Can you work these out from the drawing? Everything is in mm from the part's minimum corner. A direction names the side the tool comes from. Give positions to 0.01 mm unless a question says otherwise; leave off trailing zeros. Write each loop counter-clockwise with the first axis right and the second up, starting at its lowest first coordinate (ties: lowest second). Pieces come first, ordered by that corner, then holes. Notation, with made-up numbers: (-22.5, 34) - (-6.5, 34) arc R27 ccw to (-6.5, 65) - close; hole circle Ø8 at (-27.75, 12). An arc over 180 degrees is marked (long way). Answer in a Markdown table with one row per item.
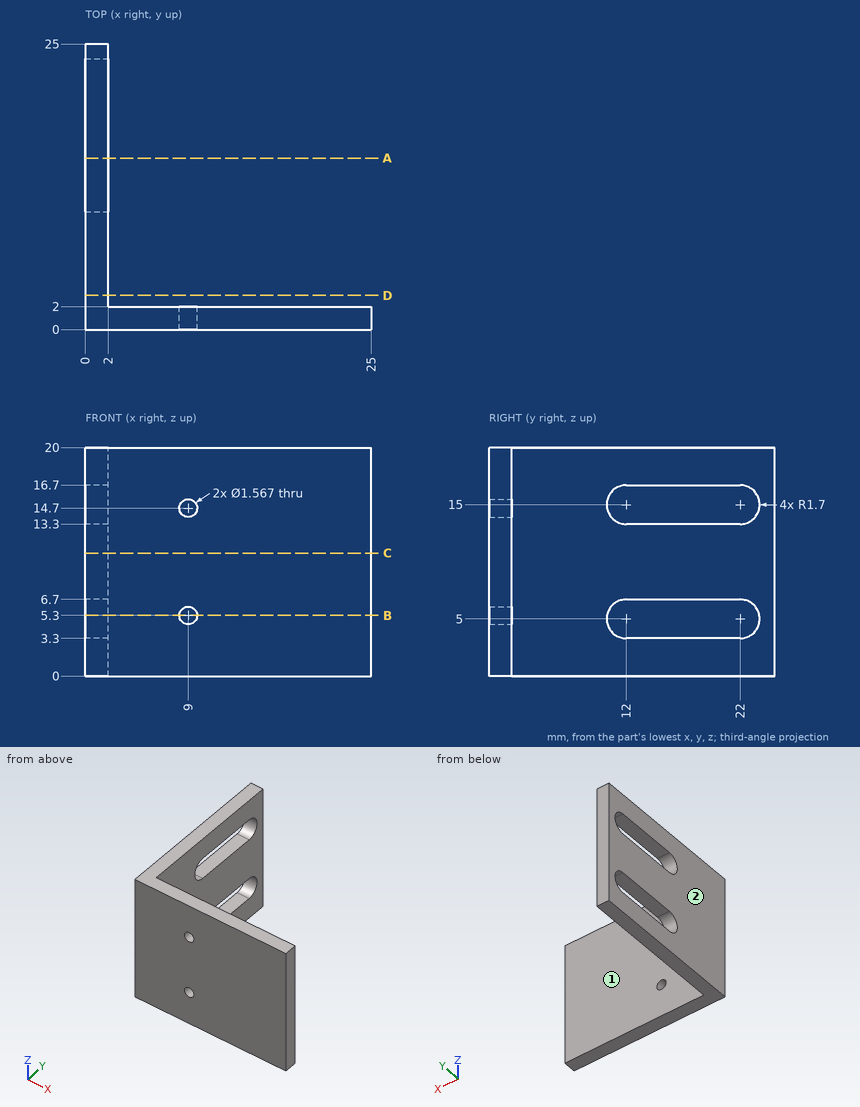
1) Will these pins go through, and if not, where does the flat tip stop? P1, Ø6, axis at x = 17.5, z = 12, coming from the +Y side; P2, Ø2, axis at x = 9, z = 5.3, coming from the -Y side; P3, Ø6, axis at y = 14, z = 6, coming from the +X side.
Check values:
| item | result |
|---|---|
| P1 | stops at y = 2 |
| P2 | stops at y = 0 |
| P3 | stops at x = 2 |
2) Imagine slicing it at B-B (z = 5.3). List the corners of the cut face in (x, y) for me, then the cut area to 3 significant figures.
Check values:
| item | result |
|---|---|
| outline | (0, 0) - (8.22, 0) - (8.22, 2) - (2, 2) - (2, 10.33) - (0, 10.33) - close; (0, 23.67) - (2, 23.67) - (2, 25) - (0, 25) - close; (9.78, 0) - (25, 0) - (25, 2) - (9.78, 2) - close |
| area | 66.2 mm2 |
3) Imagine slicing it at D-D (y = 3). List the corners of the cut face in (x, z) for me.
Check values:
| item | result |
|---|---|
| outline | (0, 0) - (2, 0) - (2, 20) - (0, 20) - close |
4) Imagine slicing it at A-A (y = 15). List the corners of the cut face in (x, z) for me.
Check values:
| item | result |
|---|---|
| outline | (0, 0) - (2, 0) - (2, 3.3) - (0, 3.3) - close; (0, 6.7) - (2, 6.7) - (2, 13.3) - (0, 13.3) - close; (0, 16.7) - (2, 16.7) - (2, 20) - (0, 20) - close |
5) If I drill on line 1 (Z direction, x = 9, y = 1.1); line 2 (X direction, y = 1.2, z = 5.3); line 3 (Y direction, x = 4.5, z = 5), over which ranges is the centre line in solid material (lowest first)?
Check values:
| item | result |
|---|---|
| line 1 | z = 0 to 4.52, 6.08 to 13.92, 15.48 to 20 |
| line 2 | x = 0 to 8.22, 9.78 to 25 |
| line 3 | y = 0 to 2 |
6) Imagine slicing it at C-C (z = 10.75). List the corners of the cut face in (x, y) for me.
Check values:
| item | result |
|---|---|
| outline | (0, 0) - (25, 0) - (25, 2) - (2, 2) - (2, 25) - (0, 25) - close |
7) On a 3-axis mill with a long thin cutter (end or side, diameter ignored), from which of +Z, -Z, +X, -X, +Y, -Y can I reach the whole of each face in a straight line? I mean the marked faces 1 and 2. Say none if no direction works.
Check values:
| item | result |
|---|---|
| face 1 | +Z, -Z, +X, +Y |
| face 2 | +Z, -Z, -X, +Y, -Y |
